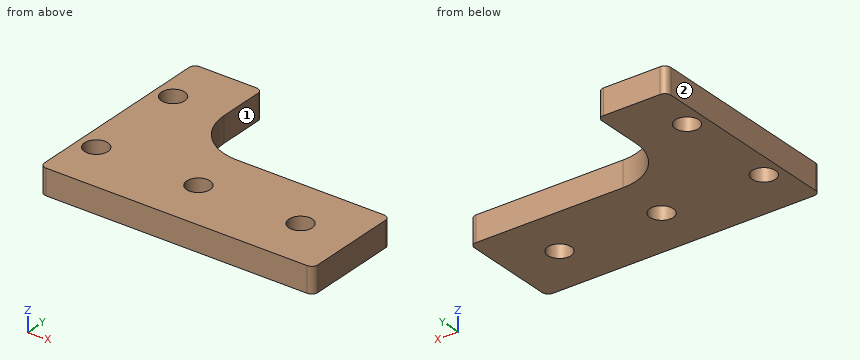
```python
from build123d import *

# Parameters (mm, degrees)
BOSS_EXTRUDE1_DEPTH = 6.35
SKETCH2_R           = 2.921
CUT_EXTRUDE1_DEPTH  = 92.800885072
SKETCH3_W           = 8.255
SKETCH3_H           = 50.8
CUT_EXTRUDE2_DEPTH  = 92.800885072
FILLET1_R           = 12.7
FILLET2_R           = 1.524


with BuildPart() as part:
    # Sketch1 → Boss-Extrude1 (new body)
    with BuildSketch(Plane.XY):
        Polygon((0, 0), (0, 50.8), (25.4, 50.8), (25.4, 25.4), (76.2, 25.4), (76.2, 0), align=None)
    extrude(amount=BOSS_EXTRUDE1_DEPTH)

    # Sketch2 → Cut-Extrude1 (cut, through all)
    with BuildSketch(Plane.XY.offset(6.35)):
        with Locations((12.7, 38.1)):
            Circle(SKETCH2_R)
        with Locations((12.7, 12.7)):
            Circle(SKETCH2_R)
        with Locations((38.1, 12.7)):
            Circle(SKETCH2_R)
        with Locations((63.5, 12.7)):
            Circle(SKETCH2_R)
    extrude(amount=-CUT_EXTRUDE1_DEPTH, mode=Mode.SUBTRACT)

    # Sketch3 → Cut-Extrude2 (cut, through all)
    with BuildSketch(Plane.XY.offset(6.35)):
        with Locations((4.1275, 25.4)):
            Rectangle(SKETCH3_W, SKETCH3_H)
    extrude(amount=-CUT_EXTRUDE2_DEPTH, mode=Mode.SUBTRACT)

    # Fillet1
    fillet1_edges = [part.edges().sort_by_distance(p)[0] for p in [
        (25.4, 25.4, 3.175),
    ]]
    fillet(fillet1_edges, radius=FILLET1_R)

    # Fillet2
    fillet2_edges = [part.edges().sort_by_distance(p)[0] for p in [
        (25.4, 50.8, 3.175),
        (76.2, 25.4, 3.175),
        (76.2, 0, 3.175),
        (8.255, 50.8, 3.175),
        (8.255, 0, 3.175),
    ]]
    fillet(fillet2_edges, radius=FILLET2_R)


solid = part.part
```
The model under review builds one solid part; all positions refer to its coordinate system, in mm. Face numbers are marked on the shaded views. A direction names the side the tool comes from. Round coordinates to 2 decimals unless told otherwise and drop trailing zeros. Write each loop counter-clockwise with the first axis right and the second up, starting at its lowest first coordinate (ties: lowest second). Pieces come first, ordered by that corner, then holes. Notation, with made-up numbers: (71, 66) - (81, 66) arc R15 cw to (81, 83) - close; hole circle Ø5 at (13.5, 15). An arc over 180 degrees is marked (long way). Answer as CSV lines item,"result". Start each with the question number.
(1) We need section A-A on x = 63.5. State the section outline as (y, z) points.
(2) We need section C-C on z = 4. State the section outline as (x, y) points (3 decimals), plus the area to 3 significant figures.
(3) We need section B-B on x = 12.7. State the section outline as (y, z) points.
(4) We need section D-D on y = 43.5. State the section outline as (x, z) points (3 decimals).
(5) For pin 1 Ø1.5 at (x, y) = (56.5, 24.5) entering from -Z; pin 2 Ø5.5 at (x, y) = (12.7, 38.1) entering from -Z; pin 3 Ø1 at (x, z) = (47.5, 2.5) entering from +Y, all flat-tipped, find the tip position at first contact; note any pin that passes through.
(6) To check wall thickness, follow line 1 (Y direction, x = 12.5, z = 0.75); line 2 (Y direction, x = 11, z = 4.5); line 3 (Y direction, x = 38.1, z = 2.5). State the ranges of each line that lie inside material, in increasing order.
(7) For the marked faces 1 and 2, list the 3-axis set-ups (+Z, -Z, +X, -X, +Y, -Y) from which the entire face can be reached by the end or side of a thin tool; tool diameter is ignored.
Worked answers:
1,outline,"(0, 0) - (9.78, 0) - (9.78, 6.35) - (0, 6.35) - close; (15.62, 0) - (25.4, 0) - (25.4, 6.35) - (15.62, 6.35) - close"
2,outline,"(8.255, 1.524) arc R1.524 ccw to (9.779, 0) - (74.676, 0) arc R1.524 ccw to (76.2, 1.524) - (76.2, 23.876) arc R1.524 ccw to (74.676, 25.4) - (38.1, 25.4) arc R12.7 cw to (25.4, 38.1) - (25.4, 49.276) arc R1.524 ccw to (23.876, 50.8) - (9.779, 50.8) arc R1.524 ccw to (8.255, 49.276) - close; hole circle Ø5.842 at (12.7, 12.7); hole circle Ø5.842 at (12.7, 38.1); hole circle Ø5.842 at (38.1, 12.7); hole circle Ø5.842 at (63.5, 12.7)"
2,area,"2,090 mm²"
3,outline,"(0, 0) - (9.78, 0) - (9.78, 6.35) - (0, 6.35) - close; (15.62, 0) - (35.18, 0) - (35.18, 6.35) - (15.62, 6.35) - close; (41.02, 0) - (50.8, 0) - (50.8, 6.35) - (41.02, 6.35) - close"
4,outline,"(8.255, 0) - (25.4, 0) - (25.4, 6.35) - (8.255, 6.35) - close"
5,pin 1,"z = 0"
5,pin 2,"through"
5,pin 3,"y = 25.4"
6,line 1,"0 to 9.79, 15.61 to 35.19, 41.01 to 50.8"
6,line 2,"0 to 10.32, 15.08 to 35.72, 40.48 to 50.8"
6,line 3,"0 to 9.78, 15.62 to 25.4"
7,face 1,"+Z, -Z, +X, +Y"
7,face 2,"+Z, -Z, -X, +Y, -Y"
